from build123d import *

# Parameters (mm, degrees)
RING_1MM_R          = 68
RING_1MM_R_2        = 63
BOSS_EXTRUDE1_DEPTH = 240
CUT_EXTRUDE2_DEPTH  = 240


with BuildPart() as part:
    # Sketch1 → Revolve1 (revolve)
    with BuildSketch(Plane(origin=(0, 0, 0), x_dir=(-1, 0, 0), z_dir=(0, 1, 0)), mode=Mode.PRIVATE) as revolve1_sk:
        Polygon((19.5, 0), (19.25, 8), (16.5, 9.5), (16.5, 20), (19.5, 20), (22, 2), (68, 2), (68, 0), align=None)
    revolve(revolve1_sk.sketch.rotate(Axis((0, 0, 20), (0, 0, -1)), 180), axis=Axis((0, 0, 20), (0, 0, -1)))

    # ring-1mm → Boss-Extrude1 (add)
    with BuildSketch(Plane.XY.offset(2)):
        Circle(RING_1MM_R)
        Circle(RING_1MM_R_2, mode=Mode.SUBTRACT)
    extrude(amount=BOSS_EXTRUDE1_DEPTH)

    # Sketch3-base-openings → Cut-Extrude2 (cut)
    with BuildSketch(Plane.XY.offset(2)):
        with BuildLine():
            Line((29.095389312, 5.13030215), (48.49231552, 8.550503583))
            ThreePointArc((48.49231552, 8.550503583), (58.682408883, 0), (48.49231552, -8.550503583))
            Line((48.49231552, -8.550503583), (29.095389312, -5.13030215))
            ThreePointArc((29.095389312, -5.13030215), (24.79055467, 0), (29.095389312, 5.13030215))
        make_face()
        with BuildLine():
            Line((27.762497352, -10.104722665), (46.27082892, -16.841204442))
            ThreePointArc((46.27082892, -16.841204442), (50.820456848, -29.341204442), (37.720325337, -31.651111078))
            Line((37.720325337, -31.651111078), (22.632195202, -18.990666647))
            ThreePointArc((22.632195202, -18.990666647), (21.469250118, -12.395277335), (27.762497352, -10.104722665))
        make_face()
        with BuildLine():
            Line((18.990666647, -22.632195202), (31.651111078, -37.720325337))
            ThreePointArc((31.651111078, -37.720325337), (29.341204442, -50.820456848), (16.841204442, -46.27082892))
            Line((16.841204442, -46.27082892), (10.104722665, -27.762497352))
            ThreePointArc((10.104722665, -27.762497352), (12.395277335, -21.469250118), (18.990666647, -22.632195202))
        make_face()
        with BuildLine():
            Line((5.13030215, -29.095389312), (8.550503583, -48.49231552))
            ThreePointArc((8.550503583, -48.49231552), (0, -58.682408883), (-8.550503583, -48.49231552))
            Line((-8.550503583, -48.49231552), (-5.13030215, -29.095389312))
            ThreePointArc((-5.13030215, -29.095389312), (0, -24.79055467), (5.13030215, -29.095389312))
        make_face()
        with BuildLine():
            Line((-10.104722665, -27.762497352), (-16.841204442, -46.27082892))
            ThreePointArc((-16.841204442, -46.27082892), (-29.341204442, -50.820456848), (-31.651111078, -37.720325337))
            Line((-31.651111078, -37.720325337), (-18.990666647, -22.632195202))
            ThreePointArc((-18.990666647, -22.632195202), (-12.395277335, -21.469250118), (-10.104722665, -27.762497352))
        make_face()
        with BuildLine():
            Line((-22.632195202, -18.990666647), (-37.720325337, -31.651111078))
            ThreePointArc((-37.720325337, -31.651111078), (-50.820456848, -29.341204442), (-46.27082892, -16.841204442))
            Line((-46.27082892, -16.841204442), (-27.762497352, -10.104722665))
            ThreePointArc((-27.762497352, -10.104722665), (-21.469250118, -12.395277335), (-22.632195202, -18.990666647))
        make_face()
        with BuildLine():
            Line((-29.095389312, -5.13030215), (-48.49231552, -8.550503583))
            ThreePointArc((-48.49231552, -8.550503583), (-58.682408883, 0), (-48.49231552, 8.550503583))
            Line((-48.49231552, 8.550503583), (-29.095389312, 5.13030215))
            ThreePointArc((-29.095389312, 5.13030215), (-24.79055467, 0), (-29.095389312, -5.13030215))
        make_face()
        with BuildLine():
            Line((-27.762497352, 10.104722665), (-46.27082892, 16.841204442))
            ThreePointArc((-46.27082892, 16.841204442), (-50.820456848, 29.341204442), (-37.720325337, 31.651111078))
            Line((-37.720325337, 31.651111078), (-22.632195202, 18.990666647))
            ThreePointArc((-22.632195202, 18.990666647), (-21.469250118, 12.395277335), (-27.762497352, 10.104722665))
        make_face()
        with BuildLine():
            Line((-18.990666647, 22.632195202), (-31.651111078, 37.720325337))
            ThreePointArc((-31.651111078, 37.720325337), (-29.341204442, 50.820456848), (-16.841204442, 46.27082892))
            Line((-16.841204442, 46.27082892), (-10.104722665, 27.762497352))
            ThreePointArc((-10.104722665, 27.762497352), (-12.395277335, 21.469250118), (-18.990666647, 22.632195202))
        make_face()
        with BuildLine():
            Line((-5.13030215, 29.095389312), (-8.550503583, 48.49231552))
            ThreePointArc((-8.550503583, 48.49231552), (0, 58.682408883), (8.550503583, 48.49231552))
            Line((8.550503583, 48.49231552), (5.13030215, 29.095389312))
            ThreePointArc((5.13030215, 29.095389312), (0, 24.79055467), (-5.13030215, 29.095389312))
        make_face()
        with BuildLine():
            Line((10.104722665, 27.762497352), (16.841204442, 46.27082892))
            ThreePointArc((16.841204442, 46.27082892), (29.341204442, 50.820456848), (31.651111078, 37.720325337))
            Line((31.651111078, 37.720325337), (18.990666647, 22.632195202))
            ThreePointArc((18.990666647, 22.632195202), (12.395277335, 21.469250118), (10.104722665, 27.762497352))
        make_face()
        with BuildLine():
            Line((22.632195202, 18.990666647), (37.720325337, 31.651111078))
            ThreePointArc((37.720325337, 31.651111078), (50.820456848, 29.341204442), (46.27082892, 16.841204442))
            Line((46.27082892, 16.841204442), (27.762497352, 10.104722665))
            ThreePointArc((27.762497352, 10.104722665), (21.469250118, 12.395277335), (22.632195202, 18.990666647))
        make_face()
    extrude(amount=-CUT_EXTRUDE2_DEPTH, mode=Mode.SUBTRACT)


solid = part.part
The model under review builds one solid part; all positions refer to its coordinate system, in mm. A direction names the side the tool comes from. Give positions to 0.01 mm unless a question says otherwise; leave off trailing zeros. Write each loop counter-clockwise with the first axis right and the second up, starting at its lowest first coordinate (ties: lowest second). Pieces come first, ordered by that corner, then holes.
1. Tool access review of faces 4 (the flat face through (15, -9, 20)), 5 (the flat face through (25.41, 30.28, 1.01)): name each direction out of +Z, -Z, +X, -X, +Y, -Y from which nothing blocks a thin tool from reaching the whole face with its end or side.
2. Add section A-A, the plane y = 0. Write out the cut boundary in (x, z), plus the area to 3 significant figures.
3. For P1, Ø12, axis at y = 35.5, z = 167.5, coming from the -X side; P2, Ø14, axis at x = -43.3, y = 25, coming from the +Z side; P3, Ø1.5, axis at x = 24.5, y = -0.5, coming from the +Z side; P4, Ø10, axis at x = 43, z = 52.5, coming from the +Y side, all flat-tipped, find the tip position at first contact; note any pin that passes through.
4. Draft analysis for pull direction X (two halves, no side actions). For faces 1 (the cylindrical face through (36.556, 57.338, 119.306)), 2 (the flat face through (60, -20, 242)), 3 (the flat face through (-37.15, -13.52, 1.01)), state which applies: +X half, -X half, draft (parallel to the pull), parting line (faces both ways), or undercut.
5. Add section B-B, the plane z = 151.5. Write out the cut boundary in (x, y), plus the area to 3 significant figures.
6. Wall thickness on L1, parallel to Y at x = -2, z = 23.5; L2, parallel to X at y = -50, z = 1; L3, parallel to X at y = -14.5, z = 72.5: over which ranges is each line inside the solid? List them lowest first.
Worked answers:
1. face 4: +Z
1. face 5: +Z, -Z
2. outline: (-68, 0) - (-58.68, 0) - (-58.68, 2) - (-63, 2) - (-63, 242) - (-68, 242) - close; (-24.79, 0) - (-19.5, 0) - (-19.25, 8) - (-16.5, 9.5) - (-16.5, 20) - (-19.5, 20) - (-22, 2) - (-24.79, 2) - close; (16.5, 9.5) - (19.25, 8) - (19.5, 0) - (24.79, 0) - (24.79, 2) - (22, 2) - (19.5, 20) - (16.5, 20) - close; (58.68, 0) - (68, 0) - (68, 242) - (63, 242) - (63, 2) - (58.68, 2) - close
2. area: 2,570 mm2
3. P1: stops at x = -61.27
3. P2: passes through
3. P3: stops at z = 2
3. P4: stops at y = 56.39
4. face 1: parting line
4. face 2: draft
4. face 3: undercut
5. outline: circle Ø136 at (0, 0); hole circle Ø126 at (0, 0)
5. area: 2,060 mm2
6. L1: y = -67.97 to -62.97, 62.97 to 67.97
6. L2: x = -46.09 to -30.52, -19.48 to -8.68, 8.68 to 19.48, 30.52 to 46.09
6. L3: x = -66.44 to -61.31, 61.31 to 66.44
